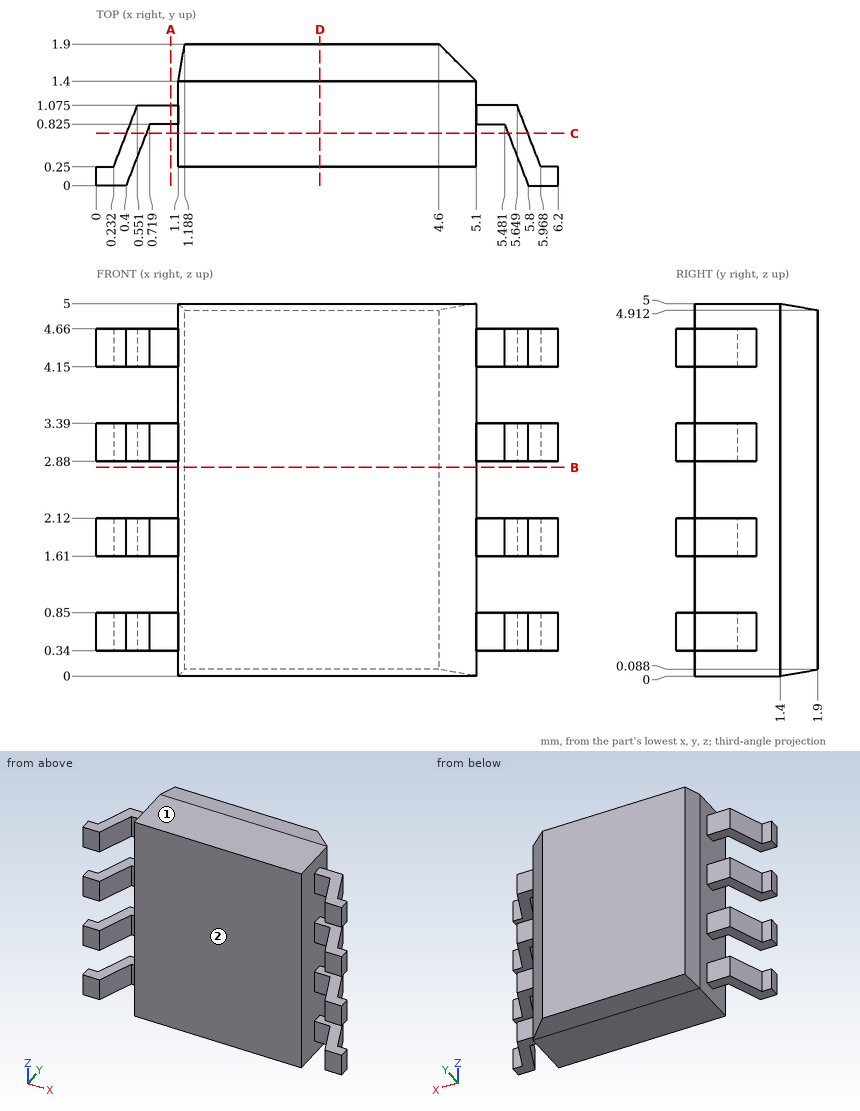
Source: three-view drawing plus pictorial views. Frame: mm from the lowest corner of the part. A direction names the side the tool comes from. Give positions to 0.01 mm unless a question says otherwise; leave off trailing zeros. Loops run counter-clockwise (first coordinate to the right, second up) from the corner with the lowest first, then second, coordinate; pieces in that order, holes last. Notation, with made-up numbers: M -27.5,-39 L -19.5,-39 A19 cw -19.5,-18 Z; hole C 52.5,64 d1. An arc over 180 degrees is marked long. Put each result on its own line as item: value.
Q1. Section B-B (z = 2.8). Return the cut outline in (x, y).
Response values:
outline: M 1.1,0.25 L 5.1,0.25 L 5.1,1.4 L 4.6,1.9 L 1.19,1.9 L 1.1,1.4 Z
Q2. Section C-C (y = 0.7). Count the separate pieces of the cut face and the enclosed holes in it, and give its area (3 significant figures).
Response values:
separate pieces: 9
enclosed holes: 0
area: 21.1 mm²
Q3. Pin query (flat end, axial travel): P1, Ø0.6, axis at x = 0.5, z = 3.5, coming from the +Y side (3 decimals); P2, Ø1, axis at x = 3.5, z = 4, coming from the -Y side; P3, Ø0.5, axis at x = 0.5, y = 0.5, coming from the -Z side. Return the tip coordinate at first contact, or that it passes through.
Response values:
P1: stops at y = 1.075
P2: stops at y = 0.25
P3: stops at z = 0.34
Q4. Section A-A (x = 1). Return the cut outline in (y, z) (3 decimals).
Response values:
outline: M 0.825,0.34 L 1.075,0.34 L 1.075,0.85 L 0.825,0.85 Z; M 0.825,1.61 L 1.075,1.61 L 1.075,2.12 L 0.825,2.12 Z; M 0.825,2.88 L 1.075,2.88 L 1.075,3.39 L 0.825,3.39 Z; M 0.825,4.15 L 1.075,4.15 L 1.075,4.66 L 0.825,4.66 Z
Q5. Section D-D (x = 3). Return the cut outline in (y, z).
Response values:
outline: M 0.25,0 L 1.4,0 L 1.9,0.09 L 1.9,4.91 L 1.4,5 L 0.25,5 Z
Q6. Reachability of the marked faces 1 and 2 from +Z, -Z, +X, -X, +Y, -Y: full face, straight path, thin tool, end or side. Return the list, or none.
Response values:
face 1: +Z, +X, -X, +Y, -Y
face 2: +Z, -Z, -Y
Q7. Line query: probe 1 along X at (y, z) = (0.3, 4.3); probe 2 along Y at (x, z) = (3.75, 2.75); probe 3 along X at (y, z) = (1.15, 0.9). Output: solid intervals per line, ascending. Write a range as [from, to].
Response values:
probe 1: x = [0.25, 0.52], [1.1, 5.1], [5.68, 5.95]
probe 2: y = [0.25, 1.9]
probe 3: x = [1.1, 5.1]
